Can you work these out from the model? Positions are in its coordinate system, mm. A direction names the side the tool comes from. Coordinates: 2 decimals unless noted, no trailing zeros. Order: outer loops, then holes, each group sorted by start corner. A loop starts at its lowest first (then second) coordinate and runs counter-clockwise, first axis right, second up. Notation, with made-up numbers: (21, -25.5) -> (35, -25.5) arc R24 ccw to (35, 8.5) -> close; hole circle Ø7 at (-30.75, -34.5). An arc over 180 degrees is marked (long way). Use a Markdown table: item, result. Add a question column.
1. For pin 1 Ø16 at (x, y) = (15, -22.5) entering from +Z; pin 2 Ø1.5 at (y, z) = (34, 74.5) entering from -X; pin 3 Ø16 at (x, y) = (12.5, -15) entering from -Z, each with a flat end and sliding along its axis, tell me the tip position at first contact or that it passes through.
2. Suppose I cut it at B-B, the plane x = 21. List the corners of the cut face in (y, z) for me.
3. Suppose I cut it at A-A, the plane y = -1. List the corners of the cut face in (x, z) for me, then the cut area to 3 significant figures.
4. We'd pull the mould along Y, two halves only. Please class faces 1 (the flat face through (-1, -50, 62)), 2 (the cylindrical face through (51, -68, 51)), 3 (the flat face through (25, 57, -2)): pulls with the +Y half, pulls with the -Y half, needs draft (parallel to the pull), parting line crosses it, or undercut.
5. For faces 4 (the flat face through (12, 1, 0)), 5 (the flat face through (25, -57, 102)), 6 (the flat face through (38, 1, 100)), which set-ups out of +Z, -Z, +X, -X, +Y, -Y let a thin tool reach every point of the face, with its end or its side?
6. Suppose I cut it at C-C, the plane z = 29. List the corners of the cut face in (x, y) for me, then the cut area to 3 significant figures.
7. If I drill on line 1 along Z through (x, y) = (42.5, -37); line 2 along X through (y, z) = (-46.5, 32); line 3 along Y through (x, z) = (49.5, 9), over which ranges is the centre line in solid material (lowest first)? Write a range as from..to.
```python
from build123d import *

# Parameters (mm, degrees)
F0_W     = 50
F0_H     = 50
F1_DEPTH = 25
F2_SIZE  = 2.5
F5_W     = 54
F5_H     = 104
F6_DEPTH = 20
F7_R     = 5


with BuildPart() as f1:
    # F0 (on Right) → F1 (new body)
    with BuildSketch(Plane.YZ):
        with Locations((25, 25)):
            Rectangle(F0_W, F0_H)
    extrude(amount=F1_DEPTH)

    # F2
    f2_edges = [f1.edges().sort_by_distance(p)[0] for p in [
        (25, 25, 50),
        (0, 25, 50),
        (25, 25, 0),
        (0, 25, 0),
    ]]
    chamfer(f2_edges, length=F2_SIZE)

    # F3: F1 across face


with BuildPart() as f1_1:
    add(f1.part)
    add(f1.part.mirror(Plane(origin=(12.5, 25, 50), x_dir=(1, 0, 0), z_dir=(0, 0, 1))))

    # F4: F1 across face


with BuildPart() as f1_2:
    add(f1_1.part)
    add(f1_1.part.mirror(Plane(origin=(25, 25, 25), x_dir=(0, 1, 0), z_dir=(1, 0, 0))))

    # F5 (on face) → F6 (join)
    with BuildSketch(Plane(origin=(0, 50, 0), x_dir=(-1, 0, 0), z_dir=(0, 1, 0))):
        with Locations((-25, 50)):
            Rectangle(F5_W, F5_H)
    extrude(amount=F6_DEPTH)

    # F7
    f7_edges = [f1_2.edges().sort_by_distance(p)[0] for p in [
        (25, 70, 102),
        (52, 70, 50),
        (25, 70, -2),
        (-2, 70, 50),
        (-2, 60, -2),
        (-2, 60, 102),
        (52, 60, 102),
        (52, 60, -2),
    ]]
    fillet(f7_edges, radius=F7_R)

    # F8: F1 across face


with BuildPart() as f1_3:
    add(f1_2.part)
    add(f1_2.part.mirror(Plane(origin=(25, 0, 50), x_dir=(1, 0, 0), z_dir=(0, -1, 0))))


solid = f1_3.part
```
Worked out:
| question | item | result |
|---|---|---|
| 1 | pin 1 | stops at z = 100 |
| 1 | pin 2 | stops at x = 0 |
| 1 | pin 3 | stops at z = 0 |
| 2 | outline | (-70, 3) arc R5 ccw to (-65, -2) -> (-50, -2) -> (-50, 0) -> (50, 0) -> (50, -2) -> (65, -2) arc R5 ccw to (70, 3) -> (70, 97) arc R5 ccw to (65, 102) -> (50, 102) -> (50, 100) -> (-50, 100) -> (-50, 102) -> (-65, 102) arc R5 ccw to (-70, 97) -> close |
| 3 | outline | (0, 2.5) -> (2.5, 0) -> (22.5, 0) -> (25, 2.5) -> (27.5, 0) -> (47.5, 0) -> (50, 2.5) -> (50, 47.5) -> (47.5, 50) -> (50, 52.5) -> (50, 97.5) -> (47.5, 100) -> (27.5, 100) -> (25, 97.5) -> (22.5, 100) -> (2.5, 100) -> (0, 97.5) -> (0, 52.5) -> (2.5, 50) -> (0, 47.5) -> close; hole (22.5, 50) -> (25, 47.5) -> (27.5, 50) -> (25, 52.5) -> close |
| 3 | area | 4,950 mm² |
| 4 | face 1 | undercut |
| 4 | face 2 | pulls with the -Y half |
| 4 | face 3 | needs draft |
| 5 | face 4 | -Z, +X, -X |
| 5 | face 5 | +Z, +X, -X, +Y, -Y |
| 5 | face 6 | +Z, +X, -X |
| 6 | outline | (-2, -65) arc R5 ccw to (3, -70) -> (47, -70) arc R5 ccw to (52, -65) -> (52, -50) -> (50, -50) -> (50, 50) -> (52, 50) -> (52, 65) arc R5 ccw to (47, 70) -> (3, 70) arc R5 ccw to (-2, 65) -> (-2, 50) -> (0, 50) -> (0, -50) -> (-2, -50) -> close |
| 6 | area | 7,140 mm² |
| 7 | line 1 | z = 0..100 |
| 7 | line 2 | x = 0..50 |
| 7 | line 3 | y = -69.33..69.33 |
